Could you check a few things on this model? Use its own coordinates, in mm. A direction names the side the tool comes from. Coordinates: 2 decimals unless noted, no trailing zeros. Loops run counter-clockwise (first coordinate to the right, second up) from the corner with the lowest first, then second, coordinate; pieces in that order, holes last.
1) If I drill on line 1 along X through (y, z) = (6, 1.2); line 2 along Y through (x, z) = (-40, 1.25); line 3 along X through (y, z) = (-8, 0.7), over which ranges is the centre line in solid material (lowest first)?
2) Will these pins go through, and if not, where does the flat tip stop? P1, Ø1, axis at x = 40.5, z = 2, coming from the +Y side; P2, Ø1, axis at x = -46.5, z = 1, coming from the +Y side; P3, Ø3, axis at x = 0, y = -67.5, coming from the -Z side; P4, Ø1.6, axis at x = -51, z = 2, coming from the -Y side.
3) Imagine slicing it at A-A on x = 0. Please give me the cut outline in (y, z) (3 decimals).
4) Thinking about a two-plate mould opening in Y: for faces 1 (the face through (55, -40, 2)), 2 (the face through (-31, 2, 2)), 3 (the face through (-1, -87.5, 2)), 4 (the face through (-37.5, -20, 1.6)), which applies, released by +Y, released by -Y, zero draft, split by the parting line, or undercut?
5) Imagine slicing it at B-B on y = -0.5. Please give me the cut outline in (x, z) (3 decimals).
6) Imagine slicing it at C-C on y = -50.5. Please give me the cut outline in (x, z) (3 decimals), plus the area to 3 significant figures.
7) For faces 5 (the face through (13, 2, 2)), 6 (the face through (-1, -18, 0)), 7 (the face through (38, 52.5, 2)), which set-ups out of +Z, -Z, +X, -X, +Y, -Y let a thin tool reach every point of the face, with its end or its side?
8) Imagine slicing it at D-D on z = 0.5. Give the number of separate pieces and of enclosed holes in the cut face, plus the area to 3 significant figures.
```python
from build123d import *

# Parameters (mm, degrees)
F0_R     = 2
F0_W     = 4
F0_H     = 11.9888
F1_DEPTH = 3.175


with BuildPart() as f1:
    # F0 (on Top) → F1 (new body)
    with BuildSketch(Plane.XY):
        with BuildLine():
            Line((-55, -57.5), (-40, -87.5))
            Line((-40, -87.5), (40, -87.5))
            Line((40, -87.5), (55, -57.5))
            Line((55, -57.5), (55, -22.5))
            Line((55, -22.5), (40, -22.5))
            Line((40, -22.5), (35, -17.5))
            Line((35, -17.5), (35, -4.123451))
            Line((35, -4.123451), (31, -4.123451))
            Line((31, -4.123451), (31, 7.865349))
            Line((31, 7.865349), (35, 7.865349))
            Line((35, 7.865349), (35, 50.876549))
            ThreePointArc((35, 50.876549), (35.475498, 52.024502), (36.623451, 52.5))
            Line((36.623451, 52.5), (40, 52.5))
            Line((40, 52.5), (45, 57.5))
            Line((45, 57.5), (55, 57.5))
            Line((55, 57.5), (55, 62.5))
            ThreePointArc((55, 62.5), (0, 87.5), (-55, 62.5))
            Line((-55, 62.5), (-55, 57.5))
            Line((-55, 57.5), (-45, 57.5))
            Line((-45, 57.5), (-40, 52.5))
            Line((-40, 52.5), (-36.623451, 52.5))
            ThreePointArc((-36.623451, 52.5), (-35.475498, 52.024502), (-35, 50.876549))
            Line((-35, 50.876549), (-35, 7.865349))
            Line((-35, 7.865349), (-31, 7.865349))
            Line((-31, 7.865349), (-31, -4.123451))
            Line((-31, -4.123451), (-35, -4.123451))
            Line((-35, -4.123451), (-35, -17.5))
            Line((-35, -17.5), (-40, -22.5))
            Line((-40, -22.5), (-55, -22.5))
            Line((-55, -22.5), (-55, -57.5))
        make_face()
        with Locations((-34, -82.5)):
            Circle(F0_R, mode=Mode.SUBTRACT)
        with Locations((-40, -50.5)):
            Circle(F0_R, mode=Mode.SUBTRACT)
        with Locations((-20, -67.5)):
            Circle(F0_R, mode=Mode.SUBTRACT)
        with Locations((0, -67.5)):
            Circle(F0_R, mode=Mode.SUBTRACT)
        with Locations((20, -67.5)):
            Circle(F0_R, mode=Mode.SUBTRACT)
        with Locations((34, -82.5)):
            Circle(F0_R, mode=Mode.SUBTRACT)
        with Locations((40, -50.5)):
            Circle(F0_R, mode=Mode.SUBTRACT)
        with Locations((0, -0.5)):
            Circle(F0_R, mode=Mode.SUBTRACT)
        with Locations((-11, 1.870949)):
            Rectangle(F0_W, F0_H, mode=Mode.SUBTRACT)
        with Locations((-40, 56.5)):
            Circle(F0_R, mode=Mode.SUBTRACT)
        with Locations((11, 1.870949)):
            Rectangle(F0_W, F0_H, mode=Mode.SUBTRACT)
        with Locations((40, 56.5)):
            Circle(F0_R, mode=Mode.SUBTRACT)
    extrude(amount=F1_DEPTH)


solid = f1.part
```
Filled in:
1. line 1: x = -31 to -13, -9 to 9, 13 to 31
1. line 2: y = -87.5 to -52.5, -48.5 to -22.5, 52.5 to 54.5, 58.5 to 75.57
1. line 3: x = -35 to 35
2. P1: stops at y = 75.57
2. P2: stops at y = 71.18
2. P3: passes through
2. P4: stops at y = -67.1
3. outline: (-87.5, 0) - (-69.5, 0) - (-69.5, 3.175) - (-87.5, 3.175) - close; (-65.5, 0) - (-2.5, 0) - (-2.5, 3.175) - (-65.5, 3.175) - close; (1.5, 0) - (87.5, 0) - (87.5, 3.175) - (1.5, 3.175) - close
4. face 1: zero draft
4. face 2: undercut
4. face 3: released by -Y
4. face 4: undercut
5. outline: (-31, 0) - (-13, 0) - (-13, 3.175) - (-31, 3.175) - close; (-9, 0) - (-2, 0) - (-2, 3.175) - (-9, 3.175) - close; (2, 0) - (9, 0) - (9, 3.175) - (2, 3.175) - close; (13, 0) - (31, 0) - (31, 3.175) - (13, 3.175) - close
6. outline: (-55, 0) - (-42, 0) - (-42, 3.175) - (-55, 3.175) - close; (-38, 0) - (38, 0) - (38, 3.175) - (-38, 3.175) - close; (42, 0) - (55, 0) - (55, 3.175) - (42, 3.175) - close
6. area: 324 mm2
7. face 5: +Z, -Z
7. face 6: -Z, +X, -X, +Y, -Y
7. face 7: +Z, -Z, +X
8. separate pieces: 1
8. enclosed holes: 12
8. area: 14,500 mm2
